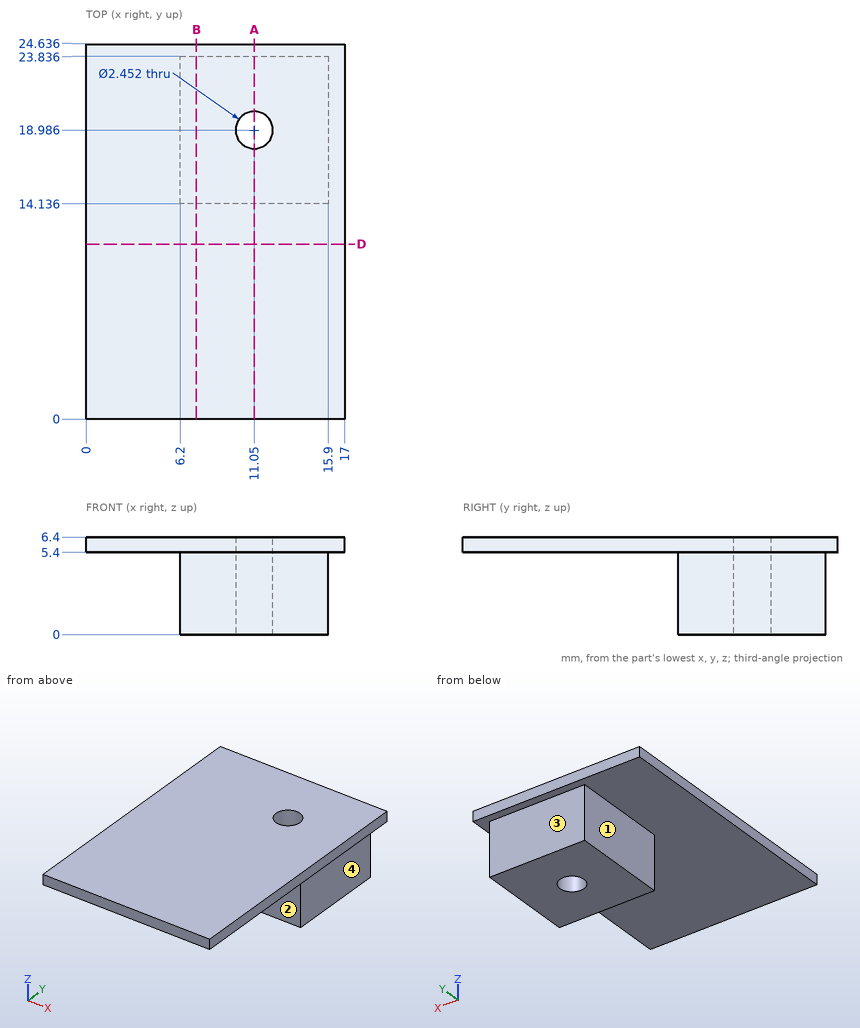
Can you work these out from the drawing? Everything is in mm from the part's minimum corner. A direction names the side the tool comes from. Give positions to 0.01 mm unless a question says otherwise; leave off trailing zeros. Loops run counter-clockwise (first coordinate to the right, second up) from the corner with the lowest first, then second, coordinate; pieces in that order, holes last. Notation, with made-up numbers: (87.5, 80) -> (142.5, 80) arc R12 cw to (142.5, 94) -> close; hole circle Ø1 at (42.5, 8.5). An arc over 180 degrees is marked (long way). Write item = value, one per line.
1) Suppose I cut it at B-B on x = 7.25. Write out the boundary of the cut face in (y, z) (1 decimal).
Check result:
outline = (0, 5.4) -> (14.1, 5.4) -> (14.1, 0) -> (23.8, 0) -> (23.8, 5.4) -> (24.6, 5.4) -> (24.6, 6.4) -> (0, 6.4) -> close
2) Suppose I cut it at D-D on y = 11.5. Write out the boundary of the cut face in (x, z).
Check result:
outline = (0, 5.4) -> (17, 5.4) -> (17, 6.4) -> (0, 6.4) -> close
3) Will these pins go through, and if not, where does the flat tip stop? pin 1 (2.5 mm diameter, centred on x = 10, z = 1.5, fed in from +Y); pin 2 (1.6 mm diameter, centred on y = 18.5, z = 1.5, fed in from +X).
Check result:
pin_1 = 23.84
pin_2 = 15.9
4) For the marked faces 1, 2, 3 and 4, which set-ups out of +Z, -Z, +X, -X, +Y, -Y let a thin tool reach every point of the face, with its end or its side?
Check result:
face_1 = -Z, -X, +Y, -Y
face_2 = -Z, +X, -X, -Y
face_3 = -Z, +X, -X, +Y
face_4 = -Z, +X, +Y, -Y
5) Suppose I cut it at A-A on x = 11.05. Write out the boundary of the cut face in (y, z) (1 decimal).
Check result:
outline = (0, 5.4) -> (14.1, 5.4) -> (14.1, 0) -> (17.8, 0) -> (17.8, 6.4) -> (0, 6.4) -> close; (20.2, 0) -> (23.8, 0) -> (23.8, 5.4) -> (24.6, 5.4) -> (24.6, 6.4) -> (20.2, 6.4) -> close
6) I need wall thicknesses on L1, parallel to X at y = 16.25, z = 1; L2, parallel to Z at x = 9.25, y = 3.5; L3, parallel to Y at x = 11.05, z = 4.5 (1 decimal). Which ranges of each line are inside material? Lowest first, please. Write a range as from..to.
Check result:
L1 = 6.2..15.9
L2 = 5.4..6.4
L3 = 14.1..17.8, 20.2..23.8
